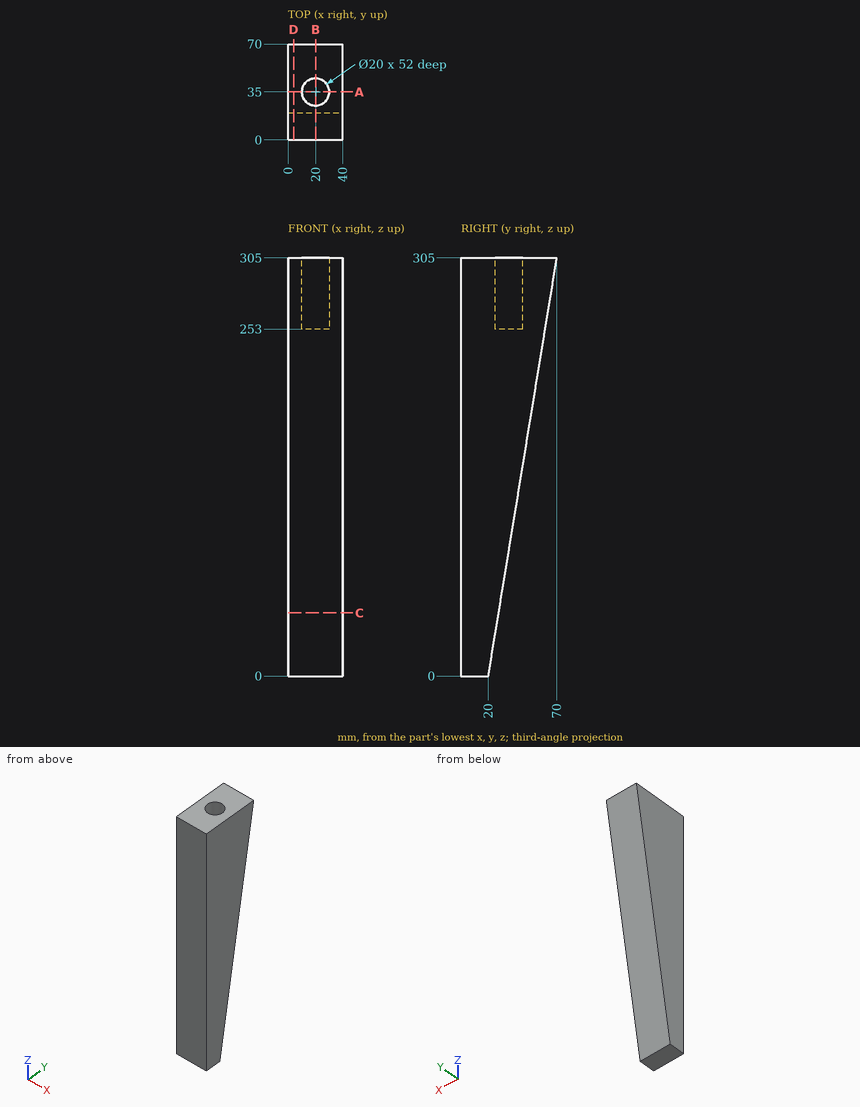
Can you work these out from the drawing? Everything is in mm from the part's minimum corner. Round coordinates to 2 decimals unless told otherwise and drop trailing zeros. Loops run counter-clockwise (first coordinate to the right, second up) from the corner with the lowest first, then second, coordinate; pieces in that order, holes last.
1. For P1, Ø16, axis at x = 20, y = 35, coming from the +Z side; P2, Ø4, axis at x = 29.5, z = 85, coming from the +Y side, each with a flat end and sliding along its axis, tell me the tip position at first contact or that it passes through.
Answer list:
P1: stops at z = 253
P2: stops at y = 34.26
2. If I drill on line 1 along X through (y, z) = (35, 292); line 2 along Y through (x, z) = (20, 281); line 3 along Y through (x, z) = (20, 274), over which ranges is the centre line in solid material (lowest first)?
Answer list:
line 1: x = 0 to 10, 30 to 40
line 2: y = 0 to 25, 45 to 66.07
line 3: y = 0 to 25, 45 to 64.92
3. If we section it at B-B on x = 20: Write out the boundary of the cut face in (y, z), plus the area to 3 significant figures.
Answer list:
outline: (0, 0) - (20, 0) - (70, 305) - (45, 305) - (45, 253) - (25, 253) - (25, 305) - (0, 305) - close
area: 12,700 mm2
4. If we section it at D-D on x = 4: Write out the boundary of the cut face in (y, z).
Answer list:
outline: (0, 0) - (20, 0) - (70, 305) - (0, 305) - close
5. If we section it at A-A on y = 35: Write out the boundary of the cut face in (x, z).
Answer list:
outline: (0, 91.5) - (40, 91.5) - (40, 305) - (30, 305) - (30, 253) - (10, 253) - (10, 305) - (0, 305) - close
6. If we section it at C-C on z = 46: Write out the boundary of the cut face in (x, y).
Answer list:
outline: (0, 0) - (40, 0) - (40, 27.54) - (0, 27.54) - close
